from build123d import *

# Parameters (mm, degrees)
SKETCH1_W           = 45.7
SKETCH1_H           = 21.3
SKETCH1_R           = 1.55
BOSS_EXTRUDE1_DEPTH = 1.2
SKETCH2_R           = 8.15
BOSS_EXTRUDE2_DEPTH = 13.3


with BuildPart() as part:
    # Sketch1 → Boss-Extrude1 (new body)
    with BuildSketch(Plane(origin=(0, 0, 0), x_dir=(1, 0, 0), z_dir=(0, 1, 0))):
        Rectangle(SKETCH1_W, SKETCH1_H)
        with Locations((20.35, 8.15)):
            Circle(SKETCH1_R, mode=Mode.SUBTRACT)
        with Locations((-20.35, -8.15)):
            Circle(SKETCH1_R, mode=Mode.SUBTRACT)
    extrude(amount=BOSS_EXTRUDE1_DEPTH)

    # Sketch2 → Boss-Extrude2 (add)
    with BuildSketch(Plane(origin=(0, 1.2, 0), x_dir=(1, 0, 0), z_dir=(0, 1, 0))):
        with Locations((-12.7, 0)):
            Circle(SKETCH2_R)
        with Locations((12.7, 0)):
            Circle(SKETCH2_R)
    extrude(amount=BOSS_EXTRUDE2_DEPTH)


solid = part.part
Input: part model. Units: mm. Frame: model coordinates. A direction names the side the tool comes from. Give positions to 0.01 mm unless a question says otherwise; leave off trailing zeros. Loops run counter-clockwise (first coordinate to the right, second up) from the corner with the lowest first, then second, coordinate; pieces in that order, holes last. Notation, with made-up numbers: (-30, -3.75) -> (3, -3.75) arc R15 cw to (3, 14.25) -> close; hole circle Ø2 at (23.25, 80.5). An arc over 180 degrees is marked (long way). Answer as a JSON object with one key per item and string values. Group by question number.
Item 1: Pin query (flat end, axial travel): P1, Ø1.5, axis at x = 0, z = -1.5, coming from the +Y side; P2, Ø4, axis at y = 7, z = 6.5, coming from the +X side; P3, Ø1, axis at y = 2, z = -3, coming from the +X side. Return the tip coordinate at first contact, or that it passes through.
Item 2: Cut plane D-D, the plane x = -11.5. Return the cut outline in (y, z).
Item 3: Pull-direction query (Z, two-part tool) for faces 1 (the flat face through (0, 1, -10.65)), 2 (the cylindrical face through (21.18, 0.59, -9.46)), 3 (the flat face through (0, 1.2, 0)); classes: released by +Z, released by -Z, zero draft, split by the parting line, or undercut.
Item 4: Cut plane B-B, the plane z = 0. Return the cut outline in (x, y), and give its area (3 significant figures).
Item 5: Cut plane A-A, the plane x = 12.7. Return the cut outline in (y, z), and give its area (3 significant figures).
Item 6: Cut plane C-C, the plane y = 11.5. Return the cut outline in (x, z).
Item 7: Line query: probe 1 along X at (y, z) = (0.9, -8.15); probe 2 along X at (y, z) = (0.4, 8.15); probe 3 along Z at (x, y) = (20.35, 0.65). Output: solid intervals per line, ascending.
Item 8: Reachability of faces 4 (the cylindrical face through (-20.842, 7.757, -0.358)), 5 (the flat face through (0, 0, 0)) from +Z, -Z, +X, -X, +Y, -Y: full face, straight path, thin tool, end or side. Return the list, or none.
Checks:
{
 "1": {"P1": "stops at y = 1.2", "P2": "stops at x = 19.5", "P3": "stops at x = 20.46"},
 "2": {"outline": "(0, -10.65) -> (1.2, -10.65) -> (1.2, -8.06) -> (14.5, -8.06) -> (14.5, 8.06) -> (1.2, 8.06) -> (1.2, 10.65) -> (0, 10.65) -> close"},
 "3": {"face 1": "released by -Z", "face 2": "undercut", "face 3": "zero draft"},
 "4": {"outline": "(-22.85, 0) -> (22.85, 0) -> (22.85, 1.2) -> (20.85, 1.2) -> (20.85, 14.5) -> (4.55, 14.5) -> (4.55, 1.2) -> (-4.55, 1.2) -> (-4.55, 14.5) -> (-20.85, 14.5) -> (-20.85, 1.2) -> (-22.85, 1.2) -> close", "area": "488 mm²"},
 "5": {"outline": "(0, -10.65) -> (1.2, -10.65) -> (1.2, -8.15) -> (14.5, -8.15) -> (14.5, 8.15) -> (1.2, 8.15) -> (1.2, 10.65) -> (0, 10.65) -> close", "area": "242 mm²"},
 "6": {"outline": "circle Ø16.3 at (-12.7, 0); circle Ø16.3 at (12.7, 0)"},
 "7": {"probe 1": "x = -22.85 to 18.8, 21.9 to 22.85", "probe 2": "x = -22.85 to -21.9, -18.8 to 22.85", "probe 3": "z = -10.65 to -9.7, -6.6 to 10.65"},
 "8": {"face 4": "+Y", "face 5": "+Z, -Z, +X, -X, -Y"}
}
